Design review of the part built by this model. Coordinates are the model's own, in mm. Face numbers are marked on the shaded views. A direction names the side the tool comes from. Coordinates: 2 decimals unless noted, no trailing zeros. Loops run counter-clockwise (first coordinate to the right, second up) from the corner with the lowest first, then second, coordinate; pieces in that order, holes last. Notation, with made-up numbers: (-21.75, 70) -> (-5.75, 70) arc R15 ccw to (-5.75, 89) -> close; hole circle Ø4 at (-33.5, 59). An arc over 180 degrees is marked (long way). Answer as a JSON object with one key per item and string values.
```python
from build123d import *

# Parameters (mm, degrees)
CUT_EXTRUDE3_DEPTH      = 186.625026901
CUT_EXTRUDE3_DEPTH_BACK = 186.625026901
SKETCH5_R               = 15
CUT_EXTRUDE4_DEPTH      = 186.017973926
CUT_EXTRUDE4_DEPTH_BACK = 186.017973926
SKETCH7_R               = 15


with BuildPart() as part:
    # Sketch2 → Revolve2 (revolve)
    with BuildSketch(Plane(origin=(0, 0, 0), x_dir=(1, 0, 0), z_dir=(0, 1, 0)), mode=Mode.PRIVATE) as revolve2_sk:
        Polygon((76.5673553, 108.935679163), (65.10595835, 63), (27.5, 63), (27.5, 43), (55, 43), (55, 35), (60, 35), (60, 0), (70, 0), (96.705505264, 107.031937471), (100, 120.235812519), (79.386848042, 120.235812519), align=None)
    revolve(revolve2_sk.sketch.rotate(Axis((0, 0, -120), (0, 0, 1)), 180), axis=Axis((0, 0, -120), (0, 0, 1)))

    # Sketch5 → Cut-Extrude3 (cut, two sides: drawn at the far end of the back side and taken through both)
    with BuildSketch(Plane(origin=(0, 0, 0), x_dir=(0, 0, -1), z_dir=(1, 0, 0)).offset(-CUT_EXTRUDE3_DEPTH_BACK)):
        with Locations((120.235812519, 0)):
            Circle(SKETCH5_R)
    extrude(amount=CUT_EXTRUDE3_DEPTH + CUT_EXTRUDE3_DEPTH_BACK, mode=Mode.SUBTRACT)

    # Sketch7 → Cut-Extrude4 (cut, two sides: drawn at the far end of the back side and taken through both)
    with BuildSketch(Plane(origin=(0, 0, 0), x_dir=(1, 0, 0), z_dir=(0, 1, 0)).offset(-CUT_EXTRUDE4_DEPTH_BACK)):
        with Locations((0, 120.235812519)):
            Circle(SKETCH7_R)
    extrude(amount=CUT_EXTRUDE4_DEPTH + CUT_EXTRUDE4_DEPTH_BACK, mode=Mode.SUBTRACT)


solid = part.part
```
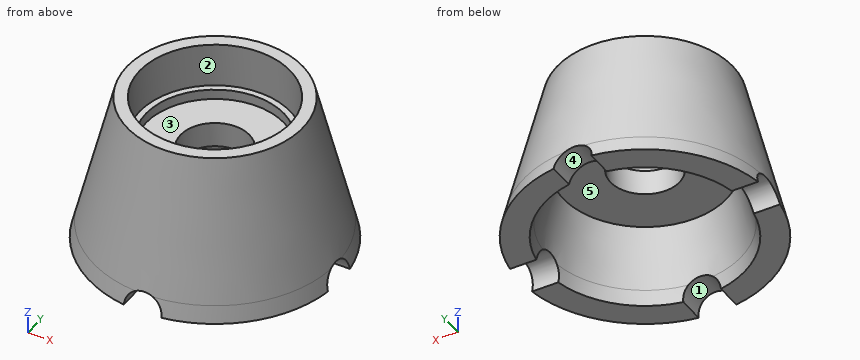
1) Wall thickness on probe 1 along Z at (x, y) = (34, 38.5); probe 2 along Y at (x, z) = (-39, -27.5); probe 3 along Y at (x, z) = (23.5, -59.5): over which ranges is each line inside the solid? List them lowest first.
Completed:
{"probe 1": "-63 to -43", "probe 2": "-66.23 to -45.6, 45.6 to 66.23", "probe 3": "-81.53 to -14.28, 14.28 to 81.53"}
2) Add section D-D, the plane z = -23. Give the boundary of the cut face in (x, y), and give its area (3 significant figures).
Completed:
{"outline": "circle Ø151.48 at (0, 0); hole circle Ø120 at (0, 0)", "area": "6,710 mm²"}
3) Add section A-A, the plane y = 0. Give the boundary of the cut face in (x, z).
Completed:
{"outline": "(-96.26, -105.24) -> (-75.64, -105.24) -> (-65.11, -63) -> (-27.5, -63) -> (-27.5, -43) -> (-55, -43) -> (-55, -35) -> (-60, -35) -> (-60, 0) -> (-70, 0) -> close; (27.5, -63) -> (65.11, -63) -> (75.64, -105.24) -> (96.26, -105.24) -> (70, 0) -> (60, 0) -> (60, -35) -> (55, -35) -> (55, -43) -> (27.5, -43) -> close"}
4) Add section C-C, the plane z = -54. Give the boundary of the cut face in (x, y), and give its area (3 significant figures).
Completed:
{"outline": "circle Ø166.95 at (0, 0); hole circle Ø55 at (0, 0)", "area": "19,500 mm²"}
5) Clearance check with flat-ended pins moving along their axes: pin 1 Ø10 at (x, z) = (10, -87.5) entering from -Y; pin 2 Ø6 at (x, y) = (21.5, -42.5) entering from -Z; pin 3 Ø6 at (x, z) = (-13.5, -63) entering from -Y. State where each tip first meets the part, or that it passes through.
Completed:
{"pin 1": "y = -92.63", "pin 2": "z = -63", "pin 3": "y = -85.53"}
6) For the marked faces 3, 4 and 5, list the 3-axis set-ups (+Z, -Z, +X, -X, +Y, -Y) from which the entire face can be reached by the end or side of a thin tool; tool diameter is ignored.
Completed:
{"face 3": "+Z", "face 4": "-Z, +Y, -Y", "face 5": "-Z"}
7) The part is to be moulded in two halves that separate along Y. For the marked faces 1 and 2, say which applies: pulls with the +Y half, pulls with the -Y half, needs draft (parallel to the pull), parting line crosses it, or undercut.
Completed:
{"face 1": "needs draft", "face 2": "undercut"}
